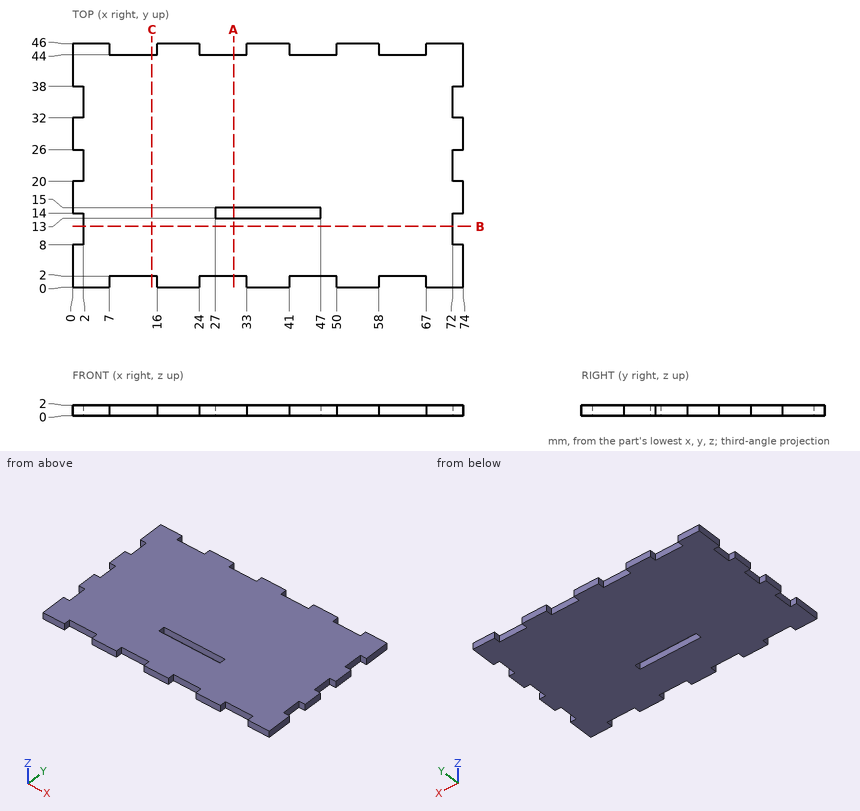
Design review of the part shown in the three views and the two pictorial views. Dimensions are in mm from the part's minimum x, y and z. Round coordinates to 2 decimals unless told otherwise and drop trailing zeros. Write each loop counter-clockwise with the first axis right and the second up, starting at its lowest first coordinate (ties: lowest second). Pieces come first, ordered by that corner, then holes.
Item 1: For pin 1 Ø1 at (x, z) = (27.5, 1) entering from -Y; pin 2 Ø1 at (y, z) = (22, 1.5) entering from +X; pin 3 Ø1 at (y, z) = (36, 1) entering from -X, all flat-tipped, find the tip position at first contact; note any pin that passes through.
Item 2: Consider section B-B on y = 11.5. Give the boundary of the cut face in (x, z), and give its area (3 significant figures).
Item 3: Consider section A-A on x = 30.5. Give the boundary of the cut face in (y, z).
Item 4: Consider section C-C on x = 15. Give the boundary of the cut face in (y, z), and give its area (3 significant figures).
Item 5: Wall thickness on L1, parallel to Y at x = 30.5, z = 1.2; L2, parallel to Y at x = 11, z = 1.7; L3, parallel to X at y = 11, z = 0.4: over which ranges is each line inside the solid? List them lowest first.
Check values:
1. pin 1: stops at y = 2
1. pin 2: stops at x = 72
1. pin 3: stops at x = 2
2. outline: (2, 0) - (72, 0) - (72, 2) - (2, 2) - close
2. area: 140 mm2
3. outline: (2, 0) - (13, 0) - (13, 2) - (2, 2) - close; (15, 0) - (44, 0) - (44, 2) - (15, 2) - close
4. outline: (2, 0) - (44, 0) - (44, 2) - (2, 2) - close
4. area: 84.0 mm2
5. L1: y = 2 to 13, 15 to 44
5. L2: y = 2 to 44
5. L3: x = 2 to 72
